from build123d import *

# Parameters (mm, degrees)
BOSS_EXTRUDE1_DEPTH = 9.55
CUT_EXTRUDE1_REACH  = 11.55
SKETCH2_R           = 2.795
SKETCH5_R           = 4.61
CUT_EXTRUDE3_DEPTH  = 5.2


with BuildPart() as part:
    # Sketch1 → Boss-Extrude1 (new body)
    with BuildSketch(Plane(origin=(0, 0, 0), x_dir=(1, 0, 0), z_dir=(0, 1, 0))):
        Polygon((532.64, 0), (545.64, 0), (545.64, -95.3), (0, -95.3), (0, 0), (92.64, 0), (92.64, -9.5), (532.64, -9.5), align=None)
    extrude(amount=BOSS_EXTRUDE1_DEPTH)

    # Sketch2 → Cut-Extrude1 (cut, up to next)
    with BuildSketch(Plane(origin=(0, 9.55, 0), x_dir=(-1, 0, 0), z_dir=(0, 1, 0)), mode=Mode.PRIVATE) as cut_extrude1_sk1:
        with Locations((-6.4, 9.38)):
            Circle(SKETCH2_R)
    cut_extrude1_tool1 = extrude(cut_extrude1_sk1.sketch, amount=-CUT_EXTRUDE1_REACH, mode=Mode.PRIVATE) & part.part
    add(cut_extrude1_tool1.solids().sort_by_distance((6.4, 9.55, 9.38))[0], mode=Mode.SUBTRACT)
    # Sketch2 → Cut-Extrude1 (cut, up to next)
    with BuildSketch(Plane(origin=(0, 9.55, 0), x_dir=(-1, 0, 0), z_dir=(0, 1, 0)), mode=Mode.PRIVATE) as cut_extrude1_sk2:
        with Locations((-6.4, 85.68)):
            Circle(SKETCH2_R)
    cut_extrude1_tool2 = extrude(cut_extrude1_sk2.sketch, amount=-CUT_EXTRUDE1_REACH, mode=Mode.PRIVATE) & part.part
    add(cut_extrude1_tool2.solids().sort_by_distance((6.4, 9.55, 85.68))[0], mode=Mode.SUBTRACT)
    # Sketch2 → Cut-Extrude1 (cut, up to next)
    with BuildSketch(Plane(origin=(0, 9.55, 0), x_dir=(-1, 0, 0), z_dir=(0, 1, 0)), mode=Mode.PRIVATE) as cut_extrude1_sk3:
        with Locations((-540.4, 85.68)):
            Circle(SKETCH2_R)
    cut_extrude1_tool3 = extrude(cut_extrude1_sk3.sketch, amount=-CUT_EXTRUDE1_REACH, mode=Mode.PRIVATE) & part.part
    add(cut_extrude1_tool3.solids().sort_by_distance((540.4, 9.55, 85.68))[0], mode=Mode.SUBTRACT)
    # Sketch2 → Cut-Extrude1 (cut, up to next)
    with BuildSketch(Plane(origin=(0, 9.55, 0), x_dir=(-1, 0, 0), z_dir=(0, 1, 0)), mode=Mode.PRIVATE) as cut_extrude1_sk4:
        with Locations((-540.4, 9.38)):
            Circle(SKETCH2_R)
    cut_extrude1_tool4 = extrude(cut_extrude1_sk4.sketch, amount=-CUT_EXTRUDE1_REACH, mode=Mode.PRIVATE) & part.part
    add(cut_extrude1_tool4.solids().sort_by_distance((540.4, 9.55, 9.38))[0], mode=Mode.SUBTRACT)

    # Sketch5 → Cut-Extrude3 (cut)
    with BuildSketch(Plane.XZ):
        with Locations((6.4, 85.68)):
            Circle(SKETCH5_R)
        with Locations((6.4, 9.38)):
            Circle(SKETCH5_R)
        with Locations((540.4, 9.38)):
            Circle(SKETCH5_R)
        with Locations((540.4, 85.68)):
            Circle(SKETCH5_R)
    extrude(amount=-CUT_EXTRUDE3_DEPTH, mode=Mode.SUBTRACT)


solid = part.part
Check sheet for the modelled part. Datum: model origin and axes. Units: mm. A direction names the side the tool comes from. Round coordinates to 2 decimals unless told otherwise and drop trailing zeros. Loops run counter-clockwise (first coordinate to the right, second up) from the corner with the lowest first, then second, coordinate; pieces in that order, holes last. Notation, with made-up numbers: M -28.75,43 L -3.75,43 A22 cw -3.75,50 Z; hole C 55.25,87.25 d10. An arc over 180 degrees is marked long. One line per question, with ' | ' between items. Start each with the question number.
Item 1: Section check B-B (x = 242). Record the boundary of the cut face in (y, z), and give its area (3 significant figures).
Item 2: Set-up check for faces 1 (the face through (0, 5, 48)), 2 (the face through (6.3, 5.2, 82.7)), 3 (the face through (532.64, 5, 5)): record each of +Z, -Z, +X, -X, +Y, -Y from which the full face is reachable in a straight line by a thin tool's end or side.
Item 3: Release check for a two-part mould opening along Z. For faces 4 (the face through (92.64, 5, 5)), 5 (the face through (5.8, 2.56, 90.25)), 6 (the face through (277, 5, 95.3)) record: released by +Z, released by -Z, zero draft, split by the parting line, or undercut.
Item 4: Section check A-A (y = 3). Record the boundary of the cut face in (x, z), and give its area (3 significant figures).
Item 5: Gauge pin test, flat ends, axial feed: pin 1 Ø6.5 at (x, z) = (540.4, 85.68) entering from -Y; pin 2 Ø7.5 at (x, z) = (8.5, 84.5) entering from -Y; pin 3 Ø4 at (x, y) = (303, 2.5) entering from -Z. Record the tip position at first contact, or that the pin passes through.
Item 6: Scan lines: probe 1 along Z at (x, y) = (540.4, 6.65) (3 decimals); probe 2 along Z at (x, y) = (6.4, 3.3); probe 3 along Z at (x, y) = (419.5, 2). Record each from-to range of solid material in increasing order.
Worked out:
1) outline: M 0,9.5 L 9.55,9.5 L 9.55,95.3 L 0,95.3 Z | area: 819 mm^2
2) face 1: +Z, -Z, -X, +Y, -Y | face 2: -Y | face 3: -Z, +Y, -Y
3) face 4: zero draft | face 5: undercut | face 6: released by +Z
4) outline: M 0,0 L 92.64,0 L 92.64,9.5 L 532.64,9.5 L 532.64,0 L 545.64,0 L 545.64,95.3 L 0,95.3 Z; hole C 6.4,9.38 d9.22; hole C 6.4,85.68 d9.22; hole C 540.4,9.38 d9.22; hole C 540.4,85.68 d9.22 | area: 47,600 mm^2
5) pin 1: y = 5.2 | pin 2: y = 0 | pin 3: z = 9.5
6) probe 1: 0 to 6.585, 12.175 to 82.885, 88.475 to 95.3 | probe 2: 0 to 4.77, 13.99 to 81.07, 90.29 to 95.3 | probe 3: 9.5 to 95.3
